Design review of the part built by this model. Coordinates are the model's own, in mm. A direction names the side the tool comes from. Give positions to 0.01 mm unless a question says otherwise; leave off trailing zeros. Loops run counter-clockwise (first coordinate to the right, second up) from the corner with the lowest first, then second, coordinate; pieces in that order, holes last.
from build123d import *

# Parameters (mm, degrees)
EXTRUDE_1_DEPTH          = 20
FILLET_1_R               = 1
CUT_EXTRUDE_1_DEPTH      = 50000
SKETCH_3_R               = 5
CUT_EXTRUDE_2_DEPTH      = 500
SKETCH_4_R               = 1.25
CUT_EXTRUDE_3_DEPTH      = 5000
PATTERN_CIRCULAR_1_COUNT = 8
SKETCH_5_R               = 3.05
SKETCH_5_R_2             = 1.5
CUT_EXTRUDE_4_DEPTH      = 5000


with BuildPart() as part:
    # 草图1 → 凸台-拉伸1 (new body)
    with BuildSketch(Plane(origin=(0, 0, 0), x_dir=(0, 0, -1), z_dir=(1, 0, 0))):
        Polygon((-24, -18.5), (-24, 16.5), (24, 16.5), (24, -18.5), (26, -18.5), (26, 18.5), (-26, 18.5), (-26, -18.5), align=None)
    extrude(amount=EXTRUDE_1_DEPTH)

    # 圆角1
    fillet_1_edges = [part.edges().sort_by_distance(p)[0] for p in [
        (10, 16.5, -24),
        (10, 16.5, 24),
        (10, 18.5, 26),
        (10, 18.5, -26),
    ]]
    fillet(fillet_1_edges, radius=FILLET_1_R)

    # 草图2 → 切除-拉伸1 (cut)
    with BuildSketch(Plane.XY.offset(26)):
        with BuildLine():
            ThreePointArc((10, -18.5), (2.928932188, -15.571067812), (0, -8.5))
            Line((0, -8.5), (0, -18.5))
            Line((0, -18.5), (10, -18.5))
        make_face()
        with BuildLine():
            ThreePointArc((20, -8.5), (17.071067812, -15.571067812), (10, -18.5))
            Line((10, -18.5), (20, -18.5))
            Line((20, -18.5), (20, -8.5))
        make_face()
    extrude(amount=-CUT_EXTRUDE_1_DEPTH, mode=Mode.SUBTRACT)

    # 草图3 → 切除-拉伸2 (cut)
    with BuildSketch(Plane.XY.offset(26)):
        with Locations((10, -8.5)):
            Circle(SKETCH_3_R)
    extrude(amount=-CUT_EXTRUDE_2_DEPTH, mode=Mode.SUBTRACT)

    # 草图4 → 切除-拉伸3 (cut)
    with BuildSketch(Plane.XY.offset(26)):
        with Locations((18, -8.5)):
            Circle(SKETCH_4_R)
    cut_extrude_3 = extrude(amount=-CUT_EXTRUDE_3_DEPTH, mode=Mode.SUBTRACT)

    # 阵列(圆周)1: 切除-拉伸3 ×8 about axis
    pattern_circular_1_axis = Axis((10, -8.5, 0), (0, 0, 1))
    for i in range(1, PATTERN_CIRCULAR_1_COUNT):
        add(cut_extrude_3.rotate(pattern_circular_1_axis, i * 360 / PATTERN_CIRCULAR_1_COUNT), mode=Mode.SUBTRACT)

    # 草图5 → 切除-拉伸4 (cut)
    with BuildSketch(Plane(origin=(0, 18.5, 0), x_dir=(1, 0, 0), z_dir=(0, 1, 0))):
        with Locations(Location((10, 0, 0), (0, 0, 270))):
            Circle(SKETCH_5_R)
        with Locations(Location((15, 15, 0), (0, 0, 270))):
            Circle(SKETCH_5_R_2)
        with Locations(Location((5, 15, 0), (0, 0, 270))):
            Circle(SKETCH_5_R_2)
        with Locations(Location((5, 5, 0), (0, 0, 270))):
            Circle(SKETCH_5_R_2)
        with Locations(Location((15, 5, 0), (0, 0, 270))):
            Circle(SKETCH_5_R_2)
        with Locations(Location((15, -5, 0), (0, 0, 270))):
            Circle(SKETCH_5_R_2)
        with Locations(Location((5, -5, 0), (0, 0, 270))):
            Circle(SKETCH_5_R_2)
        with Locations(Location((5, -15, 0), (0, 0, 270))):
            Circle(SKETCH_5_R_2)
        with Locations(Location((15, -15, 0), (0, 0, 270))):
            Circle(SKETCH_5_R_2)
    extrude(amount=-CUT_EXTRUDE_4_DEPTH, mode=Mode.SUBTRACT)


solid = part.part
Q1. Take a section at C-C (y = 2). Give the boundary of the cut face in (x, z), plus the area to 3 significant figures.
Results:
outline: (0, -26) - (20, -26) - (20, -24) - (0, -24) - close; (0, 24) - (20, 24) - (20, 26) - (0, 26) - close
area: 80.0 mm2
Q2. Take a section at A-A (x = 2). Give the boundary of the cut face in (y, z), plus the area to 3 significant figures.
Results:
outline: (-14.5, -26) - (-9.75, -26) - (-9.75, -24) - (-14.5, -24) - close; (-14.5, 24) - (-9.75, 24) - (-9.75, 26) - (-14.5, 26) - close; (-7.25, -26) - (17.5, -26) arc R1 ccw to (18.5, -25) - (18.5, 25) arc R1 ccw to (17.5, 26) - (-7.25, 26) - (-7.25, 24) - (15.5, 24) arc R1 cw to (16.5, 23) - (16.5, -23) arc R1 cw to (15.5, -24) - (-7.25, -24) - close
area: 218 mm2
Q3. Take a section at D-D (z = 15). Give the boundary of the cut face in (x, y).
Results:
outline: (0, 16.5) - (3.5, 16.5) - (3.5, 18.5) - (0, 18.5) - close; (6.5, 16.5) - (13.5, 16.5) - (13.5, 18.5) - (6.5, 18.5) - close; (16.5, 16.5) - (20, 16.5) - (20, 18.5) - (16.5, 18.5) - close
Q4. Take a section at B-B (z = 0). Give the boundary of the cut face in (x, y).
Results:
outline: (0, 16.5) - (6.95, 16.5) - (6.95, 18.5) - (0, 18.5) - close; (13.05, 16.5) - (20, 16.5) - (20, 18.5) - (13.05, 18.5) - close
Q5. Insertion check: pin 1 (5 mm diameter, centred on x = 15, z = 15, fed in from +Y); pin 2 (2 mm diameter, centred on x = 9, z = -8.5, fed in from -Y). Each pin has a flat end and moves straight along its axis. Give the tip position at first contact, or say it passes through.
Results:
pin 1: stops at y = 18.5
pin 2: stops at y = 16.5
Q6. Draft analysis for pull direction Z (two halves, no side actions). For faces 1 (the face through (5, 16.5, 0)), 2 (the face through (5.187, -3.765, -24.986)), state which applies: pulls with the +Z half, pulls with the -Z half, needs draft (parallel to the pull), parting line crosses it, or undercut.
Results:
face 1: undercut
face 2: needs draft
Q7. Tool access review of faces 3 (the face through (14.77, -7, -24.99)), 4 (the face through (10, 3, -24)): name each direction out of +Z, -Z, +X, -X, +Y, -Y from which nothing blocks a thin tool from reaching the whole face with its end or side.
Results:
face 3: +Z, -Z
face 4: +X, -X, -Y
Q8. Wall thickness on line 1 (X direction, y = 17.1, z = 15); line 2 (Z direction, x = 14.5, y = 8); line 3 (X direction, y = -8, z = 25): over which ranges is each line inside the solid? List them lowest first.
Results:
line 1: x = 0 to 3.5, 6.5 to 13.5, 16.5 to 20
line 2: z = -26 to -24, 24 to 26
line 3: x = 0 to 0.85, 3.15 to 5.03, 14.97 to 16.85, 19.15 to 20
